```python
from build123d import *

# Parameters (mm, degrees)
F0_W     = 133.35
F0_H     = 6.35
F0_H_2   = 60.325
F0_H_3   = 31.75
F0_W_2   = 6.35
F0_H_4   = 25.4
F0_H_5   = 6.8349212326
F0_H_6   = 59.8400787674
F1_DEPTH = 6.35


# Not quite as in the source:
# - a feature names something its author has since deleted; it is built from what else it names


with BuildPart() as f1:
    # F0 (on Right) → F1 (new body)
    with BuildSketch(Plane.YZ):
        with Locations((-66.675, 123.825)):
            Rectangle(F0_W, F0_H)
        with Locations((-66.675, 90.4875)):
            Rectangle(F0_W, F0_H_2)
        with Locations((66.675, 90.4875)):
            Rectangle(F0_W, F0_H_2)
        with Locations((-66.675, 44.45)):
            Rectangle(F0_W, F0_H_3)
        with Locations((-136.525, 44.45)):
            Rectangle(F0_W_2, F0_H_3)
        with Locations((66.675, 44.45)):
            Rectangle(F0_W, F0_H_3)
        with Locations((-66.675, 15.875)):
            Rectangle(F0_W, F0_H_4)
        with Locations((-142.875, 44.45)):
            Rectangle(F0_W_2, F0_H_3)
        with Locations((136.525, 44.45)):
            Rectangle(F0_W_2, F0_H_3)
        with Locations((66.675, 15.875)):
            Rectangle(F0_W, F0_H_4)
        with Locations((-66.675, -0.2424606163)):
            Rectangle(F0_W, F0_H_5)
        with Locations((-142.875, 15.875)):
            Rectangle(F0_W_2, F0_H_4)
        Polygon((146.05, 60.325), (139.7, 60.325), (139.7, 28.575), (139.7, 3.175), (146.05, 3.175), align=None)
        with Locations((-66.675, -33.5799606163)):
            Rectangle(F0_W, F0_H_6)
        with Locations((66.675, -33.5799606163)):
            Rectangle(F0_W, F0_H_6)
        with Locations((-66.675, -79.375)):
            Rectangle(F0_W, F0_H_3)
        with Locations((-136.525, -79.375)):
            Rectangle(F0_W_2, F0_H_3)
        with Locations((66.675, -79.375)):
            Rectangle(F0_W, F0_H_3)
        with Locations((-66.675, -107.95)):
            Rectangle(F0_W, F0_H_4)
        with Locations((-142.875, -79.375)):
            Rectangle(F0_W_2, F0_H_3)
        with Locations((136.525, -79.375)):
            Rectangle(F0_W_2, F0_H_3)
        with Locations((66.675, -107.95)):
            Rectangle(F0_W, F0_H_4)
        with Locations((-66.675, -123.825)):
            Rectangle(F0_W, F0_H)
        with Locations((-142.875, -107.95)):
            Rectangle(F0_W_2, F0_H_4)
        Polygon((146.05, -63.5), (139.7, -63.5), (139.7, -95.25), (139.7, -120.65), (146.05, -120.65), align=None)
    extrude(amount=F1_DEPTH)


solid = f1.part
```
The listing builds one solid part. Answer for the finished solid, in the listing's coordinates (mm). A direction names the side the tool comes from. Coordinates: 2 decimals unless noted, no trailing zeros. Write each loop counter-clockwise with the first axis right and the second up, starting at its lowest first coordinate (ties: lowest second). Pieces come first, ordered by that corner, then holes.
Q1. Which of the six approach directions +Z, -Z, +X, -X, +Y, -Y give full straight-line access (tool end or side, diameter ignored) to faces 4 (the flat face through (3, 0, -124)), 5 (the flat face through (3, -133.35, 94)), 6 (the flat face through (3, 133.35, -108)), 7 (the flat face through (3, -140, -63.5)), 8 (the flat face through (3, 133.35, 16))?
Returned:
face 4: -Z, +X, -X, +Y
face 5: +Z, +X, -X, -Y
face 6: -Z, +X, -X
face 7: +X, -X, -Y
face 8: +X, -X
Q2. Section A-A, the plane y = 15.5 is taken. Write down the section's boundary in (x, z) (3 decimals), then the cut area to 3 significant figures.
Returned:
outline: (0, -120.65) - (6.35, -120.65) - (6.35, -3.66) - (0, -3.66) - close; (0, 3.175) - (6.35, 3.175) - (6.35, 120.65) - (0, 120.65) - close
area: 1,490 mm2
Q3. Section B-B, the plane z = -111 is taken. Write down the section's boundary in (x, y), then the cut area to 3 significant figures.
Returned:
outline: (0, -146.05) - (6.35, -146.05) - (6.35, -139.7) - (0, -139.7) - close; (0, -133.35) - (6.35, -133.35) - (6.35, 133.35) - (0, 133.35) - close; (0, 139.7) - (6.35, 139.7) - (6.35, 146.05) - (0, 146.05) - close
area: 1,770 mm2
Q4. Given P1, Ø3, axis at x = 2.5, y = 138, coming from the -Z side; P2, Ø5, axis at y = -13, z = -12.5, coming from the -X side; P3, Ø1, axis at x = 5.5, z = 1.5, coming from the -Y side; P4, Ø3, axis at x = 4, z = -124.5, coming from the +Y side, each flat-ended and moving along its own axis, determine where each tip first touches the part or whether it passes through.
Returned:
P1: stops at z = -95.25
P2: stops at x = 0
P3: stops at y = -133.35
P4: stops at y = 0
Q5. Find the intervals of material crossed by line 1 along Y through (x, z) = (5.75, 17.5); line 2 along Z through (x, y) = (3.5, 118) (3 decimals); line 3 along Y through (x, z) = (3.5, -58), in increasing order.
Returned:
line 1: y = -146.05 to -139.7, -133.35 to 133.35, 139.7 to 146.05
line 2: z = -120.65 to -3.66, 3.175 to 120.65
line 3: y = -133.35 to 133.35
Q6. Section C-C, the plane z = -15.5 is taken. Write down the section's boundary in (x, y), then the cut area to 3 significant figures.
Returned:
outline: (0, -133.35) - (6.35, -133.35) - (6.35, 133.35) - (0, 133.35) - close
area: 1,690 mm2
Q7. The mould has two halves that part along Z. Classify faces 1 (the flat face through (3, 143, 3.175)), 2 (the flat face through (0, -2, 2)), 3 (the flat face through (3, -137, -95.25)): released by +Z, released by -Z, zero draft, split by the parting line, or undercut.
Returned:
face 1: undercut
face 2: zero draft
face 3: released by -Z
